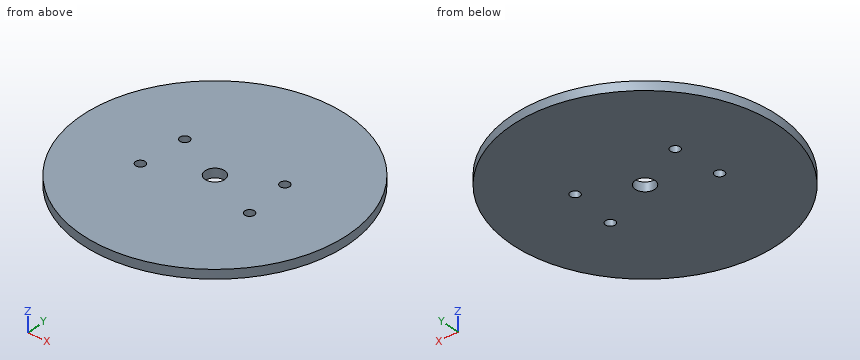
```python
from build123d import *

# Parameters (mm, degrees)
SKETCH_1_R          = 44
EXTRUDE_1_DEPTH     = 3
SKETCH_2_R          = 1.6
CUT_EXTRUDE_1_DEPTH = 3
SKETCH_3_R          = 3.25
CUT_EXTRUDE_2_DEPTH = 35


with BuildPart() as part:
    # ｽｹｯﾁ1 → ﾎﾞｽ - 押し出し1 (new body)
    with BuildSketch(Plane.XY):
        Circle(SKETCH_1_R)
    extrude(amount=EXTRUDE_1_DEPTH)

    # ｽｹｯﾁ2 → ｶｯﾄ - 押し出し1 (cut)
    with BuildSketch(Plane.XY.offset(3)):
        with Locations((-16.6, 8)):
            Circle(SKETCH_2_R)
        with Locations((-18.1, -8)):
            Circle(SKETCH_2_R)
        with Locations(Location((18.1, -8, 0), (0, 0, 180))):
            Circle(SKETCH_2_R)
        with Locations(Location((16.6, 8, 0), (0, 0, 180))):
            Circle(SKETCH_2_R)
    extrude(amount=-CUT_EXTRUDE_1_DEPTH, mode=Mode.SUBTRACT)

    # ｽｹｯﾁ3 → ｶｯﾄ - 押し出し2 (cut)
    with BuildSketch(Plane.XY.offset(3)):
        Circle(SKETCH_3_R)
    extrude(amount=-CUT_EXTRUDE_2_DEPTH, mode=Mode.SUBTRACT)


solid = part.part
```
Can you work these out from the model? Positions are in its coordinate system, mm. Give positions to 0.01 mm unless a question says otherwise; leave off trailing zeros. Write each loop counter-clockwise with the first axis right and the second up, starting at its lowest first coordinate (ties: lowest second). Pieces come first, ordered by that corner, then holes. Notation, with made-up numbers: (-16.75, 11.25) - (14.25, 11.25) arc R16 ccw to (14.25, 21.25) - close; hole circle Ø4 at (-26, 83.25). An arc over 180 degrees is marked (long way). Write item = value, one per line. Start each with the question number.
1. Please list where these lines run through material, in increasing order: line 1 (Y direction, x = 0, z = 0.7); line 2 (Y direction, x = 1, z = 2.75); line 3 (X direction, y = -24, z = 1.05).
2. Imagine slicing it at A-A (y = 0). Please give me the cut outline in (x, z).
3. For pin 1 (1.5 mm diameter, centred on x = -27.5, z = 2, fed in from +Y); pin 2 (3 mm diameter, centred on x = -16.6, y = 8, fed in from -Z), each with a flat end and sliding along its axis, tell me the tip position at first contact or that it passes through.
4. Imagine slicing it at D-D (y = -29). Please give me the cut outline in (x, z).
5. Imagine slicing it at C-C (z = 1). Please give me the cut outline in (x, y).
Worked answers:
q1.line_1 = -44 to -3.25, 3.25 to 44
q1.line_2 = -43.99 to -3.09, 3.09 to 43.99
q1.line_3 = -36.88 to 36.88
q2.outline = (-44, 0) - (-3.25, 0) - (-3.25, 3) - (-44, 3) - close; (3.25, 0) - (44, 0) - (44, 3) - (3.25, 3) - close
q3.pin_1 = 34.93
q3.pin_2 = through
q4.outline = (-33.09, 0) - (33.09, 0) - (33.09, 3) - (-33.09, 3) - close
q5.outline = circle Ø88 at (0, 0); hole circle Ø3.2 at (-18.1, -8); hole circle Ø3.2 at (-16.6, 8); hole circle Ø6.5 at (0, 0); hole circle Ø3.2 at (16.6, 8); hole circle Ø3.2 at (18.1, -8)
